Design review of the part built by this model. Coordinates are the model's own, in mm. A direction names the side the tool comes from. Round coordinates to 2 decimals unless told otherwise and drop trailing zeros. Write each loop counter-clockwise with the first axis right and the second up, starting at its lowest first coordinate (ties: lowest second). Pieces come first, ordered by that corner, then holes. Notation, with made-up numbers: M 55,68 L 71,68 A13 cw 71,92 Z; hole C 57.25,-19 d2. An arc over 180 degrees is marked long. One line per question, with ' | ' between items. Start each with the question number.
Item 1: Machinability: for faces 1 (the face through (9, 10, 5)), 2 (the face through (10.699, 0.285, 4.563)), 3 (the face through (11, 10, 4)), 4 (the face through (9.285, 19.699, 4.437)), which of the approach directions +Z, -Z, +X, -X, +Y, -Y give a long, thin tool a straight path to every point of the face, cutting with its end or side? Answer none if there is none.
Item 2: Insertion check: pin 1 Ø3 at (x, y) = (15.5, 5) entering from +Z; pin 2 Ø7 at (y, z) = (14.5, 4) entering from +X; pin 3 Ø4.5 at (y, z) = (8.5, 5) entering from -X. Each pin has a flat end and moves straight along its axis. Give the tip position at first contact, or say it passes through.
Item 3: For L1, parallel to Z at x = 15.25, y = 17; L2, parallel to X at y = 13.5, z = 4.5; L3, parallel to Z at x = 9.5, y = 14.5, list the stretches that pass through material, from the lowest coordinate up.
Item 4: Add section B-B, the plane x = 2.75. State the section outline as (y, z) points.
Autodesk Inventor part; units mm, degrees
ref_plane "YZ Plane" through (0, 0, 0) normal (1, 0, 0) x (0, 1, 0)
ref_plane "XZ Plane" through (0, 0, 0) normal (0, 1, 0) x (-1, 0, 0)
ref_plane "XY Plane" through (0, 0, 0) normal (0, 0, 1) x (1, 0, 0)
sketch "Sketch1" plane through (0, 0, 0) normal (0, 1, 0) x (-1, 0, 0)
  line L0 (0, 0) -> (-20, 0)
  line L1 (-20, 0) -> (-20, -24)
  line L2 (-20, -24) -> (0, -24)
  line L3 (0, -24) -> (0, 0)
  line L4 (-9, 0) -> (-11, 0)
  line L5 (-11, 0) -> (-11, 10)
  line L6 (-11, 10) -> (-9, 10)
  line L7 (-9, 10) -> (-9, 0)
  dimension "d0" = 20
  dimension "d1" = 24
  dimension "d2" = 2
  dimension "d3" = 10
  dimension "d4" = 9
extrude "Extrusion1" add sketch "Sketch1" along normal blind 20
fillet "Fillet1" radius 1 4 edges at (9, 20, 5) (9, 0, 5) (11, 0, 5) (11, 20, 5)
fillet "Fillet2" radius 1 4 edges at (11, 10, 10) (9.2927, 19.7073, 10) (9, 10, 10) (9.2927, 0.2927, 10)
fillet "Fillet3" radius 1 2 edges at (20, 10, 0) (0, 10, 0)
properties part number "veg_kapcs_erzekelo_meretezett"
Computed values:
1) face 1: +Z, -X, +Y, -Y | face 2: +Z, +X, -Y | face 3: +Z, +X, +Y, -Y | face 4: +Z, -X, +Y
2) pin 1: stops at z = 0 | pin 2: stops at x = 11 | pin 3: stops at x = 9
3) L1: z = -24 to 0 | L2: x = 9 to 11 | L3: z = -24 to 9.87
4) outline: M 0,-24 L 20,-24 L 20,0 L 0,0 Z
